Part print with two shaded views. Sizes in mm from the minimum x, y, z corner. Give positions to 0.01 mm unless a question says otherwise; leave off trailing zeros. Write each loop counter-clockwise with the first axis right and the second up, starting at its lowest first coordinate (ties: lowest second). Pieces come first, ordered by that corner, then holes.
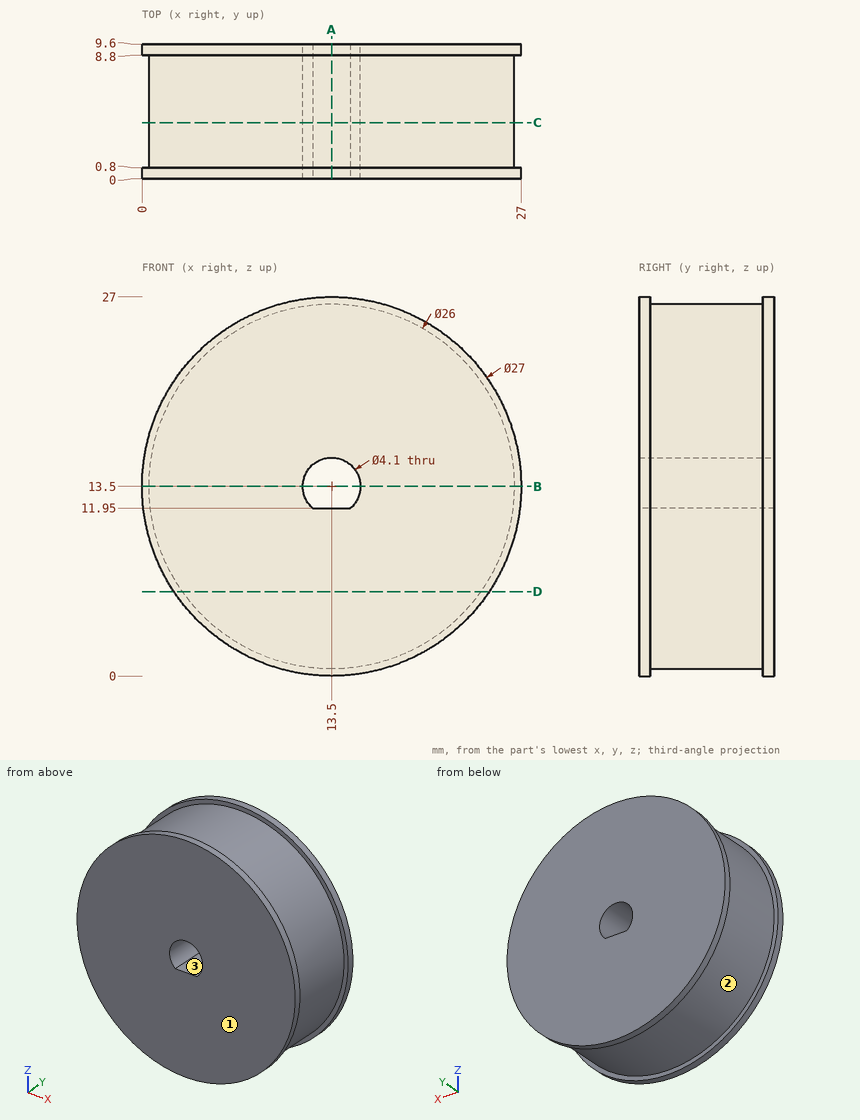
1) Mould opens along X. For the marked faces 1, 2 and 3 say: +X half, -X half, draft (parallel to the pull), parting line (faces both ways), or undercut.
Check result:
face 1: draft
face 2: parting line
face 3: undercut
2) Saw through at A-A (x = 13.5). Write the cut outline in (y, z), and give its area (3 significant figures).
Check result:
outline: (0, 0) - (0.8, 0) - (0.8, 0.5) - (8.8, 0.5) - (8.8, 0) - (9.6, 0) - (9.6, 11.95) - (0, 11.95) - close; (0, 15.55) - (9.6, 15.55) - (9.6, 27) - (8.8, 27) - (8.8, 26.5) - (0.8, 26.5) - (0.8, 27) - (0, 27) - close
area: 217 mm2
3) Saw through at D-D (z = 6). Write the cut outline in (x, y), and give its area (3 significant figures).
Check result:
outline: (2.28, 0) - (24.72, 0) - (24.72, 0.8) - (24.12, 0.8) - (24.12, 8.8) - (24.72, 8.8) - (24.72, 9.6) - (2.28, 9.6) - (2.28, 8.8) - (2.88, 8.8) - (2.88, 0.8) - (2.28, 0.8) - close
area: 206 mm2
4) Saw through at C-C (y = 4). Write the cut outline in (x, z).
Check result:
outline: circle Ø26 at (13.5, 13.5); hole (12.16, 11.95) - (14.84, 11.95) arc R2.05 ccw (long way) to start
5) Flat gauge pins, fed straight in: P1, Ø3, axis at y = 1, z = 20.5, coming from the +X side; P2, Ø2, axis at x = 14, y = 3, coming from the +Z side; P3, Ø2, axis at y = 4.5, z = 11, coming from the -X side. Where does each tip first touch, or does it go through?
Check result:
P1: stops at x = 25.82
P2: stops at z = 26.5
P3: stops at x = 0.59
6) Drill centre lines: L1, parallel to X at y = 4.75, z = 13.5; L2, parallel to Z at x = 14, y = 5; L3, parallel to X at y = 4, z = 15. Where is each one in solid material? Low to high.
Check result:
L1: x = 0.5 to 11.45, 15.55 to 26.5
L2: z = 0.51 to 11.95, 15.49 to 26.49
L3: x = 0.59 to 12.1, 14.9 to 26.41
7) Saw through at B-B (z = 13.5). Write the cut outline in (x, y).
Check result:
outline: (0, 0) - (11.45, 0) - (11.45, 9.6) - (0, 9.6) - (0, 8.8) - (0.5, 8.8) - (0.5, 0.8) - (0, 0.8) - close; (15.55, 0) - (27, 0) - (27, 0.8) - (26.5, 0.8) - (26.5, 8.8) - (27, 8.8) - (27, 9.6) - (15.55, 9.6) - close
